Here's how the part is built. I have some questions about the finished solid (model axes, mm). A direction names the side the tool comes from. Round coordinates to 2 decimals unless told otherwise and drop trailing zeros. Write each loop counter-clockwise with the first axis right and the second up, starting at its lowest first coordinate (ties: lowest second). Pieces come first, ordered by that corner, then holes. Notation, with made-up numbers: (29.25, 55.5) - (54.25, 55.5) arc R28 cw to (54.25, 83.5) - close; hole circle Ø10 at (39, 67.5). An arc over 180 degrees is marked (long way). Return JSON: item names as keys, results as strings. Group by question number.
```python
from build123d import *

# Parameters (mm, degrees)
SKETCH1_W           = 60
SKETCH1_H           = 30
BOSS_EXTRUDE1_DEPTH = 5
SKETCH6_R           = 6.374885251
SKETCH6_R_2         = 3.302926723
BOSS_EXTRUDE5_DEPTH = 20


with BuildPart() as part:
    # Sketch1 → Boss-Extrude1 (new body)
    with BuildSketch(Plane.XY):
        with Locations((30, -15)):
            Rectangle(SKETCH1_W, SKETCH1_H)
    extrude(amount=BOSS_EXTRUDE1_DEPTH)

    # Sketch6 → Boss-Extrude5 (add)
    with BuildSketch(Plane.ZY.offset(-20)):
        with Locations((0, 3.924359496)):
            Circle(SKETCH6_R)
        with Locations((0, 3.924359496)):
            Circle(SKETCH6_R_2, mode=Mode.SUBTRACT)
    extrude(amount=-BOSS_EXTRUDE5_DEPTH)


solid = part.part
```
1) Will these pins go through, and if not, where does the flat tip stop? pin 1 Ø15 at (x, y) = (31, -8.5) entering from -Z; pin 2 Ø3 at (y, z) = (5.5, -1.5) entering from -X; pin 3 Ø4 at (y, z) = (6, 1.5) entering from +X; pin 4 Ø5 at (y, z) = (-19.5, -2) entering from +X.
2) Imagine slicing it at D-D (x = 46). Please give me the cut outline in (y, z), plus the area to 3 significant figures.
3) Imagine slicing it at B-B (x = 25.5). Please give me the cut outline in (y, z).
4) Imagine slicing it at C-C (y = -22.5). Please give me the cut outline in (x, z).
5) For faces 1 (the flat face through (0, -15, 2)), 2 (the flat face through (50, 0, 2)), 3 (the flat face through (10, 0, 2)), which set-ups out of +Z, -Z, +X, -X, +Y, -Y let a thin tool reach every point of the face, with its end or its side?
6) If we mould it in two halves opening along Z, with no side actions, what happens to faces 4 (the flat face through (30, -15, 5)), 5 (the flat face through (30, -15, 0)), 6 (the cylindrical face through (29.86, 0.7, -0.72)), 7 (the flat face through (60, -15, 2))? For each: released by +Z, released by -Z, zero draft, split by the parting line, or undercut.
7) I need wall thicknesses on line 1 along Z through (x, y) = (31, -15); line 2 along X through (y, z) = (8, 4); line 3 along Y through (x, z) = (8, 0.25). Which ranges of each line are inside material? Lowest first, please.
8) Imagine slicing it at A-A (z = 2.5). Please give me the cut outline in (x, y), plus the area to 3 significant figures.
Results found:
{
 "1": {"pin 1": "stops at z = -4.05", "pin 2": "stops at x = 20", "pin 3": "stops at x = 40", "pin 4": "stops at x = 60"},
 "2": {"outline": "(-30, 0) - (0, 0) - (0, 5) - (-30, 5) - close", "area": "150 mm²"},
 "3": {"outline": "(-30, 0) - (-2.45, 0) arc R6.37 ccw (long way) to (-0.03, 5) - (-30, 5) - close; hole circle Ø6.61 at (3.92, 0)"},
 "4": {"outline": "(0, 0) - (60, 0) - (60, 5) - (0, 5) - close"},
 "5": {"face 1": "+Z, -Z, -X, +Y, -Y", "face 2": "+Z, -Z, +X, +Y", "face 3": "+Z, -Z, -X, +Y"},
 "6": {"face 4": "released by +Z", "face 5": "released by -Z", "face 6": "undercut", "face 7": "zero draft"},
 "7": {"line 1": "z = 0 to 5", "line 2": "x = 20 to 40", "line 3": "y = -30 to 0"},
 "8": {"outline": "(0, -30) - (60, -30) - (60, 0) - (40, 0) - (40, 1.77) - (20, 1.77) - (20, 0) - (0, 0) - close; (20, 6.08) - (40, 6.08) - (40, 9.79) - (20, 9.79) - close", "area": "1,910 mm²"}
}
